```python
from build123d import *

# Parameters (mm, degrees)
BOSS_EXTRUDE2_DEPTH = 187.452
CUT_EXTRUDE1_DEPTH  = 186.182
FILLET1_R           = 2.54
FILLET2_R           = 2.54


with BuildPart() as part:
    # Sketch2 → Boss-Extrude2 (new body)
    with BuildSketch(Plane(origin=(0, 0, 0), x_dir=(0, 0, -1), z_dir=(1, 0, 0))):
        Polygon((31.75, 18.330871047), (-31.75, 18.330871047), (0, -36.661742094), align=None)
    extrude(amount=BOSS_EXTRUDE2_DEPTH)

    # Sketch3 → Cut-Extrude1 (cut)
    with BuildSketch(Plane(origin=(0, 0, 0), x_dir=(0, 0, -1), z_dir=(1, 0, 0))):
        Polygon((30.1625, 17.414327494), (-30.1625, 17.414327494), (0, -34.828654989), align=None)
    extrude(amount=CUT_EXTRUDE1_DEPTH, mode=Mode.SUBTRACT)

    # Fillet1
    fillet1_edges = [part.edges().sort_by_distance(p)[0] for p in [
        (93.091, -34.828654989, 0),
        (93.091, 17.414327494, -30.1625),
        (93.091, 17.414327494, 30.1625),
        (93.726, -36.661742094, 0),
        (93.726, 18.330871047, 31.75),
        (93.726, 18.330871047, -31.75),
    ]]
    fillet(fillet1_edges, radius=FILLET1_R)

    # Fillet2
    fillet2_edges = [part.edges().sort_by_distance(p)[0] for p in [
        (186.182, -8.707163747, 15.08125),
        (186.182, -8.707163747, -15.08125),
        (186.182, 17.414327494, 0),
        (186.182, 16.144327494, -27.962795474),
        (186.182, 16.144327494, 27.962795474),
        (186.182, -32.288654989, 0),
        (187.452, -9.165435523, -15.875),
        (187.452, -9.165435523, 15.875),
        (187.452, 18.330871047, 0),
        (187.452, 17.060871047, -29.550295474),
        (187.452, 17.060871047, 29.550295474),
        (187.452, -34.121742094, 0),
    ]]
    fillet(fillet2_edges, radius=FILLET2_R)


solid = part.part
```
Check sheet for the modelled part. Datum: model origin and axes. Units: mm. A direction names the side the tool comes from. Give positions to 0.01 mm unless a question says otherwise; leave off trailing zeros. Order: outer loops, then holes, each group sorted by start corner. A loop starts at its lowest first (then second) coordinate and runs counter-clockwise, first axis right, second up. Notation, with made-up numbers: M -21.75,-2.5 L 8.25,-2.5 A30 cw 8.25,21.5 Z; hole C -8,54 d5. An arc over 180 degrees is marked long. Answer in a Markdown table with one row per item.
1) Cross-section at A-A, the plane x = 115. Enter the section's corners in (y, z), plus the area to 3 significant figures.
Filled sheet:
| item | result |
|---|---|
| outline | M -32.85,-2.2 L 14.52,-29.55 A2.54 ccw 18.33,-27.35 L 18.33,27.35 A2.54 ccw 14.52,29.55 L -32.85,2.2 A2.54 ccw Z; hole M -31.02,-2.2 L 13.6,-27.96 A2.54 ccw 17.41,-25.76 L 17.41,25.76 A2.54 ccw 13.6,27.96 L -31.02,2.2 A2.54 ccw Z |
| area | 170 mm2 |
2) Thickness scan on L1, parallel to X at y = -18, z = -4.5; L2, parallel to Y at x = 18.5, z = -9; L3, parallel to Y at x = 13, z = 2.5. Record the ranges inside material, lowest first. Write a range as [from, to].
Filled sheet:
| item | result |
|---|---|
| L1 | x = [186.18, 187.45] |
| L2 | y = [-21.07, -19.24], [17.41, 18.33] |
| L3 | y = [-32.33, -30.5], [17.41, 18.33] |
3) Release check for a two-part mould opening along Y. For faces 1 (the flat face through (91, 18.331, 0)), 2 (the cylindrical face through (93.11, -32.29, 0.04)), 3 (the cylindrical face through (186.728, -9.115, 15.022)) record: +Y half, -Y half, draft (parallel to the pull), parting line (faces both ways), or undercut.
Filled sheet:
| item | result |
|---|---|
| face 1 | +Y half |
| face 2 | undercut |
| face 3 | -Y half |
4) Access from +Z, -Z, +X, -X, +Y, -Y to the whole of each face (thin tool, end or side, straight path). Record for faces 4 (the flat face through (90.54, -9.02, -14.9)), 5 (the cylindrical face through (93.75, -34.12, -0.04)).
Filled sheet:
| item | result |
|---|---|
| face 4 | -X |
| face 5 | +X, -X, -Y |
5) Gauge pin test, flat ends, axial feed: P1, Ø6, axis at x = 52, z = -22.5, coming from the -Y side; P2, Ø1, axis at x = 95.5, y = -17.5, coming from the -Z side; P3, Ø2, axis at x = 112, y = -20, coming from the +Z side. Record the tip position at first contact, or that the pin passes through.
Filled sheet:
| item | result |
|---|---|
| P1 | stops at y = -2.89 |
| P2 | stops at z = -11.35 |
| P3 | stops at z = 10.2 |
